```python
from build123d import *

# Parameters (mm, degrees)
BOSS_EXTRUDE1_DEPTH = 1.8
CUT_EXTRUDE2_REACH  = 3.8
BOSS_EXTRUDE2_DEPTH = 1.8
BOSS_EXTRUDE3_DEPTH = 6.4
CUT_EXTRUDE3_REACH  = 10.2
SKETCH7_R           = 1.45


with BuildPart() as part:
    # Sketch1 → Boss-Extrude1 (new body)
    with BuildSketch(Plane(origin=(0, 0, 0), x_dir=(1, 0, 0), z_dir=(0, 1, 0))):
        Polygon((0, 15), (0, 0), (17, 0), (17, 10), align=None)
    extrude(amount=BOSS_EXTRUDE1_DEPTH)

    # Sketch3 → Cut-Extrude2 (cut, up to next)
    with BuildSketch(Plane(origin=(0, 1.8, 0), x_dir=(1, 0, 0), z_dir=(0, 1, 0)), mode=Mode.PRIVATE) as cut_extrude2_sk1:
        with BuildLine():
            Line((0, 15), (0, 5.504405832))
            add(Edge.make_bspline(
                [(17, 3.138617849), (8.707332044, 5.198817795), (0, 5.504405832)],
                knots=[4.238740022, 4.238740022, 4.238740022, 4.471680234, 4.471680234, 4.471680234], degree=2, weights=[1, 0.993225021, 1]))
            Line((17, 3.138617849), (17, 10))
            Line((17, 10), (0, 15))
        make_face()
    cut_extrude2_tool1 = extrude(cut_extrude2_sk1.sketch, amount=-CUT_EXTRUDE2_REACH, mode=Mode.PRIVATE) & part.part
    add(cut_extrude2_tool1.solids().sort_by_distance((8.024676, 1.8, -8.663074))[0], mode=Mode.SUBTRACT)

    # Sketch5 → Boss-Extrude2 (add)
    with BuildSketch(Plane(origin=(0, 1.8, 0), x_dir=(1, 0, 0), z_dir=(0, 1, 0))):
        Polygon((17, 0), (17, -18), (2.5e-08, -18), (0, 0), align=None)
    extrude(amount=-BOSS_EXTRUDE2_DEPTH)

    # Sketch6 → Boss-Extrude3 (add)
    with BuildSketch(Plane.XZ):
        Polygon((2.5e-08, 18), (17, 18), (17, 12.4), (1.9e-08, 12.4), align=None)
    extrude(amount=BOSS_EXTRUDE3_DEPTH)

    # Sketch7 → Cut-Extrude3 (cut, up to next)
    with BuildSketch(Plane(origin=(0, 1.8, 0), x_dir=(1, 0, 0), z_dir=(0, 1, 0)), mode=Mode.PRIVATE) as cut_extrude3_sk1:
        with Locations(Location((8.500000012, -15, 0), (0, 0, 270))):  # turned: the seam where the file's is
            Circle(SKETCH7_R)
    cut_extrude3_tool1 = extrude(cut_extrude3_sk1.sketch, amount=-CUT_EXTRUDE3_REACH, mode=Mode.PRIVATE) & part.part
    add(cut_extrude3_tool1.solids().sort_by_distance((8.5, 1.8, 15))[0], mode=Mode.SUBTRACT)


solid = part.part
```
Geometry: final body of the model. Coordinates: model frame, mm. A direction names the side the tool comes from. Coordinates: 2 decimals unless noted, no trailing zeros. Order: outer loops, then holes, each group sorted by start corner. A loop starts at its lowest first (then second) coordinate and runs counter-clockwise, first axis right, second up. Notation, with made-up numbers: (-18, -17.5) -> (-5, -17.5) arc R22 cw to (-5, -11.5) -> close; hole circle Ø4 at (7, 8). An arc over 180 degrees is marked (long way). Answer in a Markdown table with one row per item.
Item 1: Draft query along X for faces 3 (the cylindrical face through (8.94, -2.24, 16.38)), 4 (the flat face through (17, 0.5, 12.3)), 5 (the flat face through (9, 0, 3)). Return one class per face: released by +X, released by -X, zero draft, split by the parting line, or undercut.
Return value:
| item | result |
|---|---|
| face 3 | undercut |
| face 4 | released by +X |
| face 5 | zero draft |
Item 2: Section B-B on y = -4.25. Output: boundary loops of the cut face in (x, z), plus the area to 3 significant figures.
Return value:
| item | result |
|---|---|
| outline | (0, 12.4) -> (17, 12.4) -> (17, 18) -> (0, 18) -> close; hole circle Ø2.9 at (8.5, 15) |
| area | 88.6 mm² |
Item 3: Access query for faces 1 (the flat face through (9, -3, 12.4)), 2 (the flat face through (9, -6.4, 17)). Directions: +Z, -Z, +X, -X, +Y, -Y. A direction counts if a zero-diameter tool reaches every point of the face in a straight line with its end or side. Return the directions, or none.
Return value:
| item | result |
|---|---|
| face 1 | -Z, +X, -X, -Y |
| face 2 | +Z, -Z, +X, -X, -Y |
Item 4: Ray query, L1, parallel to X at y = -3.25, z = 15; L2, parallel to Z at x = 4.5, y = -5; L3, parallel to Y at x = 4, z = -3. Return the intervals inside material, ascending.
Return value:
| item | result |
|---|---|
| L1 | x = 0 to 7.05, 9.95 to 17 |
| L2 | z = 12.4 to 18 |
| L3 | y = 0 to 1.8 |
Item 5: Section C-C on z = 1.5. Output: boundary loops of the cut face in (x, y).
Return value:
| item | result |
|---|---|
| outline | (0, 0) -> (17, 0) -> (17, 1.8) -> (0, 1.8) -> close |
Item 6: Section A-A on z = 15. Output: boundary loops of the cut face in (x, y).
Return value:
| item | result |
|---|---|
| outline | (0, -6.4) -> (7.05, -6.4) -> (7.05, 1.8) -> (0, 1.8) -> close; (9.95, -6.4) -> (17, -6.4) -> (17, 1.8) -> (9.95, 1.8) -> close |
Item 7: Contact query for flat-ended pins moving along their axis: P1, Ø3.5, axis at x = 8.5, z = 15, coming from the -Y side; P2, Ø3, axis at x = 9, y = -3.5, coming from the -Z side. Output: stop coordinate, or through.
Return value:
| item | result |
|---|---|
| P1 | stops at y = -6.4 |
| P2 | stops at z = 12.4 |
